Design review of the part built by this model. Coordinates are the model's own, in mm. Face numbers are marked on the shaded views. Coordinates: 2 decimals unless noted, no trailing zeros. Write each loop counter-clockwise with the first axis right and the second up, starting at its lowest first coordinate (ties: lowest second). Pieces come first, ordered by that corner, then holes. Notation, with made-up numbers: M 75.5,80 L 108.5,80 A14 ccw 108.5,95 Z; hole C -2.5,-16.5 d1. An arc over 180 degrees is marked long. One line per question, with ' | ' between items.
from build123d import *

# Parameters (mm, degrees)
SKETCH_1_R      = 1.5
SKETCH_1_R_2    = 5
EXTRUDE_1_DEPTH = 3


with BuildPart() as part:
    # 草图1 → 凸台-拉伸1 (new body)
    with BuildSketch(Plane.XY):
        with BuildLine():
            Line((-2.598076211, 21.5), (-19.918584287, -8.5))
            ThreePointArc((-19.918584287, -8.5), (-19.918584287, -11.5), (-17.320508076, -13))
            Line((-17.320508076, -13), (17.320508076, -13))
            ThreePointArc((17.320508076, -13), (19.918584287, -11.5), (19.918584287, -8.5))
            Line((19.918584287, -8.5), (2.598076211, 21.5))
            ThreePointArc((2.598076211, 21.5), (0, 23), (-2.598076211, 21.5))
        make_face()
        with Locations((-17.320508076, -10)):
            Circle(SKETCH_1_R, mode=Mode.SUBTRACT)
        with Locations((0, 20)):
            Circle(SKETCH_1_R, mode=Mode.SUBTRACT)
        with Locations((17.320508076, -10)):
            Circle(SKETCH_1_R, mode=Mode.SUBTRACT)
        Circle(SKETCH_1_R_2, mode=Mode.SUBTRACT)
        with Locations((0, 7)):
            Circle(SKETCH_1_R, mode=Mode.SUBTRACT)
        with Locations((0, -7)):
            Circle(SKETCH_1_R, mode=Mode.SUBTRACT)
    extrude(amount=EXTRUDE_1_DEPTH)


solid = part.part
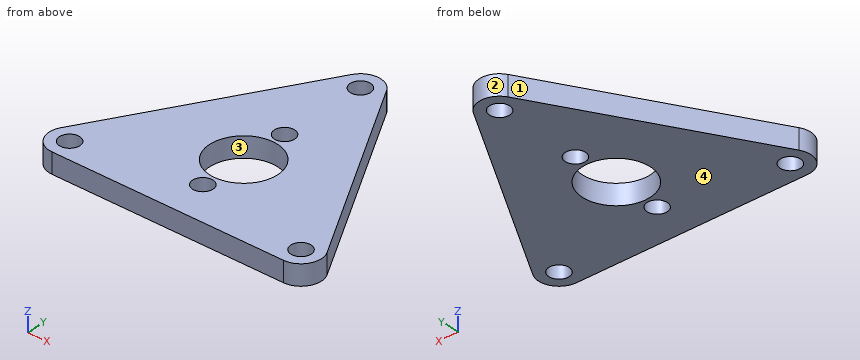
1. Take a section at D-D (y = 2.5). Write out the cut boundary in (x, z), then the cut area to 3 significant figures.
Answer sheet:
outline: M -13.57,0 L -4.33,0 L -4.33,3 L -13.57,3 Z; M 4.33,0 L 13.57,0 L 13.57,3 L 4.33,3 Z | area: 55.4 mm^2
2. To check wall thickness, follow line 1 along Y through (x, z) = (0, 2); line 2 along Y through (x, z) = (1, 1.9); line 3 along X through (y, z) = (-2, 2.8). State the ranges of each line that lie inside material, in increasing order. Write a range as [from, to].
Answer sheet:
line 1: [-13, -8.5], [-5.5, -5], [5, 5.5], [8.5, 18.5], [21.5, 23] | line 2: [-13, -8.12], [-5.88, -4.9], [4.9, 5.88], [8.12, 18.88], [21.12, 22.83] | line 3: [-16.17, -4.58], [4.58, 16.17]
3. Draft analysis for pull direction X (two halves, no side actions). For the marked faces 1, 2, 3 and 4, state which applies: pulls with the +X half, pulls with the -X half, needs draft (parallel to the pull), parting line crosses it, or undercut.
Answer sheet:
face 1: pulls with the -X half | face 2: parting line crosses it | face 3: undercut | face 4: needs draft
4. Take a section at A-A (x = 0). Write out the cut boundary in (y, z), then the cut area to 3 significant figures.
Answer sheet:
outline: M -13,0 L -8.5,0 L -8.5,3 L -13,3 Z; M -5.5,0 L -5,0 L -5,3 L -5.5,3 Z; M 5,0 L 5.5,0 L 5.5,3 L 5,3 Z; M 8.5,0 L 18.5,0 L 18.5,3 L 8.5,3 Z; M 21.5,0 L 23,0 L 23,3 L 21.5,3 Z | area: 51.0 mm^2
5. Take a section at C-C (z = 0.55). Write out the cut boundary in (x, y), then the cut area to 3 significant figures.
Answer sheet:
outline: M -19.92,-8.5 A3 ccw -17.32,-13 L 17.32,-13 A3 ccw 19.92,-8.5 L 2.6,21.5 A3 ccw -2.6,21.5 Z; hole C -17.32,-10 d3; hole C 0,0 d10; hole C 0,-7 d3; hole C 0,7 d3; hole C 0,20 d3; hole C 17.32,-10 d3 | area: 746 mm^2
6. Take a section at B-B (y = -10). Write out the cut boundary in (x, z), then the cut area to 3 significant figures.
Answer sheet:
outline: M -20.32,0 L -18.82,0 L -18.82,3 L -20.32,3 Z; M -15.82,0 L 15.82,0 L 15.82,3 L -15.82,3 Z; M 18.82,0 L 20.32,0 L 20.32,3 L 18.82,3 Z | area: 104 mm^2
